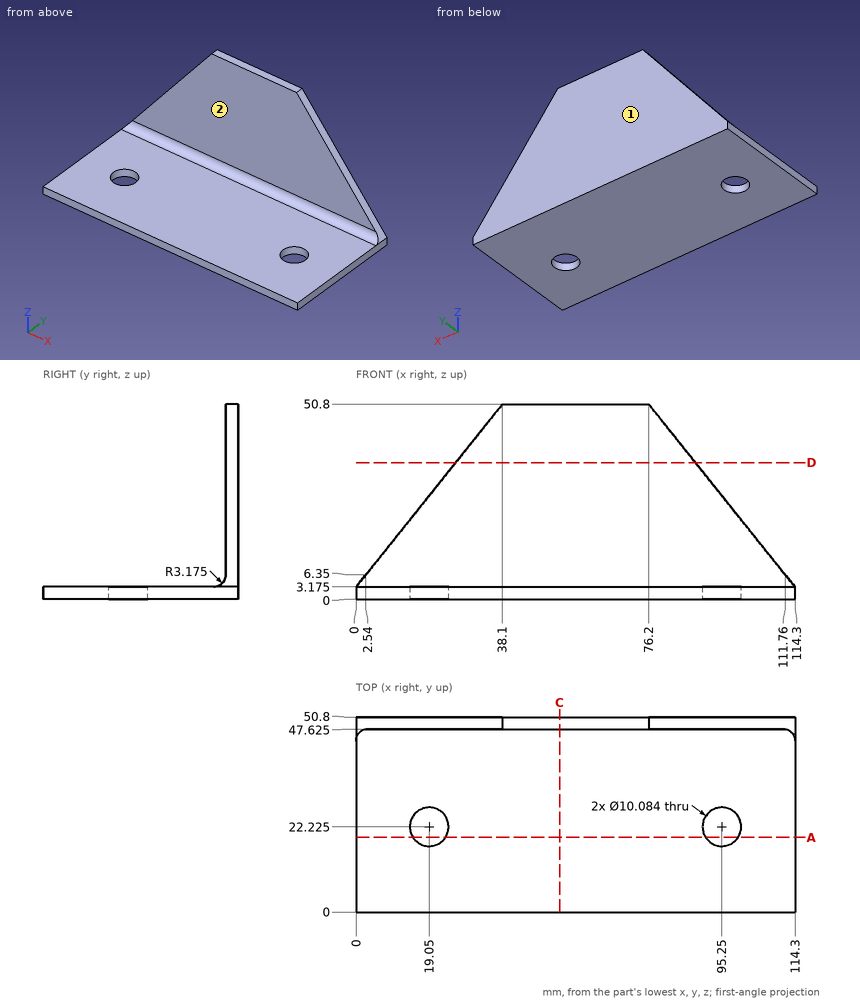
For this review, use the dimensioned drawing (mm, ordinates from the lowest corner) and the shaded views. A direction names the side the tool comes from. Coordinates: 2 decimals unless noted, no trailing zeros. Loops run counter-clockwise (first coordinate to the right, second up) from the corner with the lowest first, then second, coordinate; pieces in that order, holes last. Notation, with made-up numbers: (-14.75, 48) - (33.25, 48) arc R23 cw to (33.25, 82) - close; hole circle Ø2 at (15, -16). An arc over 180 degrees is marked (long way). Use CSV: the item, a comma, the result in double quotes. Start each with the question number.
1) Consider section C-C on x = 53. Write out the cut boundary in (y, z) (3 decimals).
2) For pin 1 Ø10 at (x, y) = (47.5, 39) entering from +Z (3 decimals); pin 2 Ø22 at (x, z) = (71, 21.5) entering from -Y (3 decimals); pin 3 Ø4 at (x, y) = (80.5, 44) entering from +Z, all flat-tipped, find the tip position at first contact; note any pin that passes through.
3) Consider section D-D on z = 35.5. Write out the cut boundary in (x, y) (3 decimals).
4) Consider section A-A on y = 19.5. Write out the cut boundary in (x, z) (3 decimals), then the cut area to 3 significant figures.
5) Wall thickness on L1, parallel to Z at x = 71.5, y = 39.5 (3 decimals); L2, parallel to Y at x = 28, z = 20 (3 decimals); L3, parallel to Z at x = 85, y = 46: over which ranges is each line inside the solid? List them lowest first. Write a range as from..to.
6) Tool access review of the marked faces 1 and 2: name each direction out of +Z, -Z, +X, -X, +Y, -Y from which nothing blocks a thin tool from reaching the whole face with its end or side.
Geometry says:
1,outline,"(0, 0) - (50.8, 0) - (50.8, 50.8) - (47.625, 50.8) - (47.625, 6.35) arc R3.175 cw to (44.45, 3.175) - (0, 3.175) - close"
2,pin 1,"z = 3.175"
2,pin 2,"y = 47.625"
2,pin 3,"z = 3.58"
3,outline,"(25.86, 47.625) - (88.44, 47.625) - (88.44, 50.8) - (25.86, 50.8) - close"
4,outline,"(0, 0) - (14.808, 0) - (14.808, 3.175) - (0, 3.175) - close; (23.292, 0) - (91.008, 0) - (91.008, 3.175) - (23.292, 3.175) - close; (99.492, 0) - (114.3, 0) - (114.3, 3.175) - (99.492, 3.175) - close"
4,area,"309 mm^2"
5,L1,"0..3.175"
5,L2,"47.625..50.8"
5,L3,"0..3.58"
6,face 1,"+Z, -Z, +X, -X, +Y"
6,face 2,"+Z, +X, -X, -Y"
